Autodesk Inventor part; units mm, degrees
ref_plane "YZ Plane" through (0, 0, 0) normal (1, 0, 0) x (0, 1, 0)
ref_plane "XZ Plane" through (0, 0, 0) normal (0, 1, 0) x (-1, 0, 0)
ref_plane "XY Plane" through (0, 0, 0) normal (0, 0, 1) x (1, 0, 0)
sketch "Sketch1" plane through (0, 0, 0) normal (0, 0, 1) x (1, 0, 0)
  line L0 (3.6662, 6.35) -> (7.3323, 0)
  line L1 (7.3323, 0) -> (3.6662, -6.35)
  line L2 (3.6662, -6.35) -> (-3.6662, -6.35)
  line L3 (-3.6662, -6.35) -> (-7.3323, 0)
  line L4 (-7.3323, 0) -> (-3.6662, 6.35)
  line L5 (-3.6662, 6.35) -> (3.6662, 6.35)
  circle A0 centre (0, 0) radius 19.05
  dimension "d0" = 12.7
  dimension "d1" = 38.1
extrude "Extrusion1" add sketch "Sketch1" along normal mid plane 1.5875
properties part number "SPACER,HEX,INTAKE" material "Nylon 6/6"
The listing builds one solid part. Answer for the finished solid, in the listing's coordinates (mm). A direction names the side the tool comes from. Round coordinates to 2 decimals unless told otherwise and drop trailing zeros. Write each loop counter-clockwise with the first axis right and the second up, starting at its lowest first coordinate (ties: lowest second). Pieces come first, ordered by that corner, then holes. Notation, with made-up numbers: (-26.75, -24.75) -> (29.25, -24.75) arc R16 cw to (29.25, -16.75) -> close; hole circle Ø11 at (4, 62). An arc over 180 degrees is marked (long way). Write item = value, one per line.
1) Which of the six approach directions +Z, -Z, +X, -X, +Y, -Y give full straight-line access (tool end or side, diameter ignored) to faces 1 (the flat face through (8, 0, 0.794)), 2 (the flat face through (-5.474, -3.219, 0.011))?
Check values:
face_1 = +Z, +X, -X, +Y, -Y
face_2 = +Z, -Z
2) Section B-B on y = 2 is taken. Write down the section's boundary in (x, z), plus the area to 3 significant figures.
Check values:
outline = (-18.94, -0.79) -> (-6.18, -0.79) -> (-6.18, 0.79) -> (-18.94, 0.79) -> close; (6.18, -0.79) -> (18.94, -0.79) -> (18.94, 0.79) -> (6.18, 0.79) -> close
area = 40.5 mm²
3) Section D-D on y = -16 is taken. Write down the section's boundary in (x, z).
Check values:
outline = (-10.34, -0.79) -> (10.34, -0.79) -> (10.34, 0.79) -> (-10.34, 0.79) -> close
4) For a pull along Y with two mould halves and no side action, classify faces 3 (the cylindrical face through (-15.12, 11.59, -0.01)), 4 (the flat face through (5.474, 3.219, -0.011)), 5 (the flat face through (8, 0, -0.794)) as released by +Y, released by -Y, zero draft, split by the parting line, or undercut.
Check values:
face_3 = split by the parting line
face_4 = undercut
face_5 = zero draft
5) Section C-C on z = 0.3 is taken. Write down the section's boundary in (x, y).
Check values:
outline = circle Ø38.1 at (0, 0); hole (-7.33, 0) -> (-3.67, -6.35) -> (3.67, -6.35) -> (7.33, 0) -> (3.67, 6.35) -> (-3.67, 6.35) -> close
6) Straight lines are drawn through the part: line 1 along Y through (x, z) = (0, -0.4); line 2 along X through (y, z) = (3, 0); line 3 along X through (y, z) = (2.5, 0.2). For each, find the intervals that lie inside material, in ascending order. Write a range as [from, to].
Check values:
line_1 = [-19.05, -6.35], [6.35, 19.05]
line_2 = [-18.81, -5.6], [5.6, 18.81]
line_3 = [-18.89, -5.89], [5.89, 18.89]
7) Given pin 1 (0.5 mm diameter, centred on x = -1.5, z = 0, fed in from -Y); pin 2 (0.8 mm diameter, centred on x = -1, z = 0.5, fed in from +Y), each flat-ended and moving along its own axis, determine where each tip first touches the part or whether it passes through.
Check values:
pin_1 = -19.01
pin_2 = 19.04
8) Section A-A on x = 0 is taken. Write down the section's boundary in (y, z).
Check values:
outline = (-19.05, -0.79) -> (-6.35, -0.79) -> (-6.35, 0.79) -> (-19.05, 0.79) -> close; (6.35, -0.79) -> (19.05, -0.79) -> (19.05, 0.79) -> (6.35, 0.79) -> close
